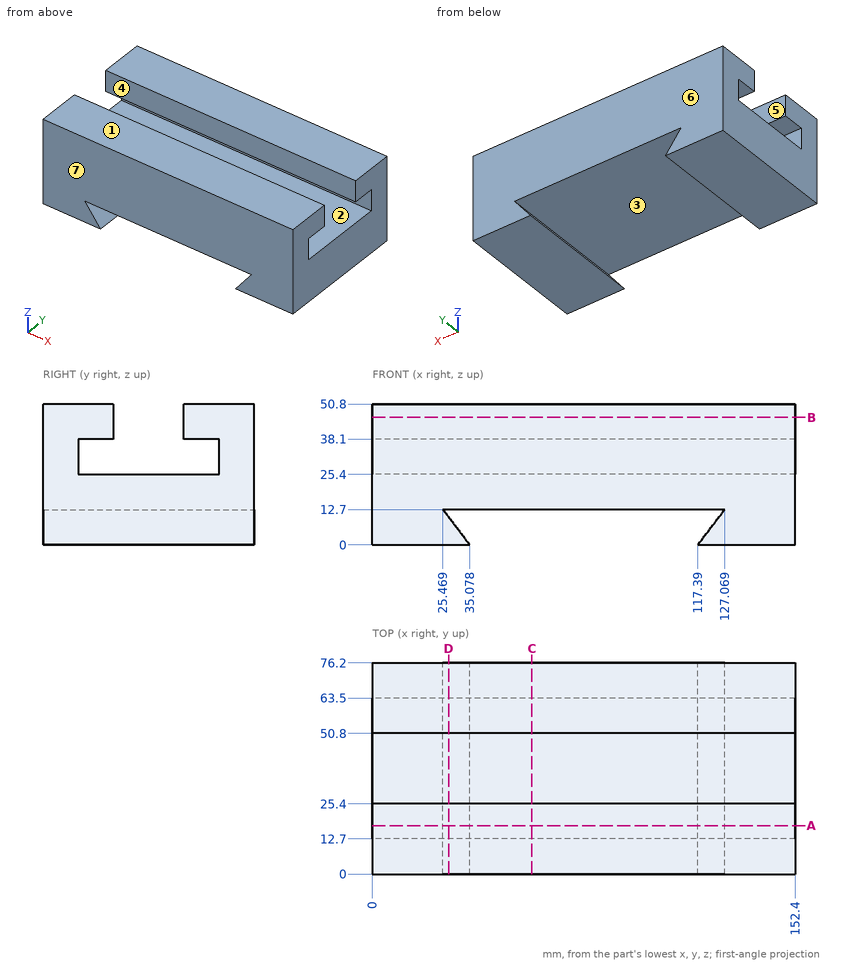
Geometry check sheet. Reference: drawing and pictorial views, mm from the part's lowest x, y, z. A direction names the side the tool comes from. Round coordinates to 2 decimals unless told otherwise and drop trailing zeros. Order: outer loops, then holes, each group sorted by start corner. A loop starts at its lowest first (then second) coordinate and runs counter-clockwise, first axis right, second up.
Q1. Set-up check for the marked faces 1, 2, 3 and 4: record each of +Z, -Z, +X, -X, +Y, -Y from which the full face is reachable in a straight line by a thin tool's end or side.
Filled sheet:
face 1: +Z, +X, -X, +Y, -Y
face 2: +X, -X
face 3: +Y, -Y
face 4: +Z, +X, -X
Q2. Scan lines: L1, parallel to Y at x = 46, z = 42; L2, parallel to Y at x = 109, z = 37; L3, parallel to Z at x = 80.5, y = 23.5. Record each from-to range of solid material in increasing order.
Filled sheet:
L1: y = 0 to 25.4, 50.8 to 76.2
L2: y = 0 to 12.7, 63.5 to 76.2
L3: z = 12.7 to 25.4, 38.1 to 50.8
Q3. Depth check by flat-ended pin: P1, Ø4, axis at x = 43, y = 54, coming from the -Z side. Enter the tip coordinate at first touch or a pass-through.
Filled sheet:
P1: stops at z = 12.7
Q4. Cross-section at C-C, the plane x = 57.5. Enter the section's corners in (y, z), plus the area to 3 significant figures.
Filled sheet:
outline: (0, 12.7) - (76.2, 12.7) - (76.2, 50.8) - (50.8, 50.8) - (50.8, 38.1) - (63.5, 38.1) - (63.5, 25.4) - (12.7, 25.4) - (12.7, 38.1) - (25.4, 38.1) - (25.4, 50.8) - (0, 50.8) - close
area: 1,940 mm2
Q5. Cross-section at B-B, the plane z = 46. Enter the section's corners in (x, y).
Filled sheet:
outline: (0, 0) - (152.4, 0) - (152.4, 25.4) - (0, 25.4) - close; (0, 50.8) - (152.4, 50.8) - (152.4, 76.2) - (0, 76.2) - close
Q6. Cross-section at D-D, the plane x = 27.5. Enter the section's corners in (y, z) (1 decimal), plus the area to 3 significant figures.
Filled sheet:
outline: (0, 0) - (76.2, 0) - (76.2, 10) - (0, 10) - close; (0, 12.7) - (76.2, 12.7) - (76.2, 50.8) - (50.8, 50.8) - (50.8, 38.1) - (63.5, 38.1) - (63.5, 25.4) - (12.7, 25.4) - (12.7, 38.1) - (25.4, 38.1) - (25.4, 50.8) - (0, 50.8) - close
area: 2,700 mm2
Q7. Draft check along Y on the marked faces 5, 6 and 7. Enter one of: pulls with the +Y half, pulls with the -Y half, needs draft (parallel to the pull), parting line crosses it, or undercut.
Filled sheet:
face 5: undercut
face 6: pulls with the +Y half
face 7: pulls with the -Y half
Q8. Cross-section at A-A, the plane y = 17.5. Enter the section's corners in (x, z), plus the area to 3 significant figures.
Filled sheet:
outline: (0, 0) - (35.08, 0) - (25.47, 12.7) - (127.07, 12.7) - (117.39, 0) - (152.4, 0) - (152.4, 25.4) - (0, 25.4) - close; (0, 38.1) - (152.4, 38.1) - (152.4, 50.8) - (0, 50.8) - close
area: 4,640 mm2
